from build123d import *

# Parameters (mm, degrees)
SKETCH1_W           = 81.5
SKETCH1_H           = 35
BOSS_EXTRUDE1_DEPTH = 3
SKETCH2_W           = 81.5
SKETCH2_H           = 35
BOSS_EXTRUDE2_DEPTH = 25.5


with BuildPart() as part:
    # Sketch1 → Boss-Extrude1 (new body)
    with BuildSketch(Plane(origin=(0, 0, 0), x_dir=(1, 0, 0), z_dir=(0, 1, 0))):
        with Locations((40.75, 17.5)):
            Rectangle(SKETCH1_W, SKETCH1_H)
    extrude(amount=BOSS_EXTRUDE1_DEPTH)

    # Sketch2 → Boss-Extrude2 (add)
    with BuildSketch(Plane(origin=(0, 3, 0), x_dir=(1, 0, 0), z_dir=(0, 1, 0))):
        with Locations((40.75, 17.5)):
            Rectangle(SKETCH2_W, SKETCH2_H)
        Polygon((79, 5), (79, 6.25), (77.899410911, 6.25), (77.899410911, 7.5), (79, 7.5), (79, 8.75), (77.899410911, 8.75), (77.899410911, 10), (79, 10), (79, 11.25), (77.899410911, 11.25), (77.899410911, 12.5), (79, 12.5), (79, 13.75), (77.899410911, 13.75), (77.899410911, 15), (79, 15), (79, 16.25), (77.899410911, 16.25), (77.899410911, 17.5), (79, 17.5), (79, 18.75), (77.899410911, 18.75), (77.899410911, 20), (79, 20), (79, 21.25), (77.899410911, 21.25), (77.899410911, 22.5), (79, 22.5), (79, 23.75), (77.899410911, 23.75), (77.899410911, 25), (79, 25), (79, 26.25), (77.899410911, 26.25), (77.899410911, 27.5), (79, 27.5), (79, 28.75), (77.899410911, 28.75), (77.899410911, 30), (79, 30), (79, 31.25), (77.899410911, 31.25), (77.899410911, 32.5), (3.600589089, 32.5), (3.600589089, 31.25), (2.5, 31.25), (2.5, 30), (3.600589089, 30), (3.600589089, 28.75), (2.5, 28.75), (2.5, 27.5), (3.600589089, 27.5), (3.600589089, 26.25), (2.5, 26.25), (2.5, 25), (3.600589089, 25), (3.600589089, 23.75), (2.5, 23.75), (2.5, 22.5), (3.600589089, 22.5), (3.600589089, 21.25), (2.5, 21.25), (2.5, 20), (3.600589089, 20), (3.600589089, 18.75), (2.5, 18.75), (2.5, 17.5), (3.600589089, 17.5), (3.600589089, 16.25), (2.5, 16.25), (2.5, 15), (3.600589089, 15), (3.600589089, 13.75), (2.5, 13.75), (2.5, 12.5), (3.600589089, 12.5), (3.600589089, 11.25), (2.5, 11.25), (2.5, 10), (3.600589089, 10), (3.600589089, 8.75), (2.5, 8.75), (2.5, 7.5), (3.600589089, 7.5), (3.600589089, 6.25), (2.5, 6.25), (2.5, 5), (3.600589089, 5), (3.600589089, 3.75), (2.5, 3.75), (2.5, 2.5), (79, 2.5), (79, 3.75), (77.899410911, 3.75), (77.899410911, 5), align=None, mode=Mode.SUBTRACT)
    extrude(amount=BOSS_EXTRUDE2_DEPTH)


solid = part.part
Could you check a few things on this model? Use its own coordinates, in mm. A direction names the side the tool comes from. Give positions to 0.01 mm unless a question says otherwise; leave off trailing zeros. Loops run counter-clockwise (first coordinate to the right, second up) from the corner with the lowest first, then second, coordinate; pieces in that order, holes last. Notation, with made-up numbers: M 51,71 L 89,71 A29 cw 89,93 Z; hole C 53.5,64.25 d4. An arc over 180 degrees is marked long. Answer as a JSON object with one key per item and string values.
Q1. If we mould it in two halves opening along X, with no side actions, what happens to faces 3 (the flat face through (81.5, 14, -17)), 4 (the flat face through (40, 16, -2.5)), 5 (the flat face through (40, 0, -18))? For each: pulls with the +X half, pulls with the -X half, needs draft (parallel to the pull), parting line crosses it, or undercut.
Values found:
{"face 3": "pulls with the +X half", "face 4": "undercut", "face 5": "needs draft"}
Q2. For P1, Ø8, axis at x = 61.5, z = -8, coming from the +Y side, with a flat end and sliding along its axis, tell me the tip position at first contact or that it passes through.
Values found:
{"P1": "stops at y = 3"}
Q3. If I drill on probe 1 along Z at (x, y) = (50.5, 22); probe 2 along X at (y, z) = (6.5, -20.5); probe 3 along Y at (x, z) = (15, -19.5), over which ranges is the centre line in solid material (lowest first)? Write a range as [from, to].
Values found:
{"probe 1": "z = [-35, -32.5], [-2.5, 0]", "probe 2": "x = [0, 2.5], [79, 81.5]", "probe 3": "y = [0, 3]"}
Q4. For faces 1 (the flat face through (41, 16, -32.5)), 2 (the flat face through (0, 14, -17)), which set-ups out of +Z, -Z, +X, -X, +Y, -Y let a thin tool reach every point of the face, with its end or its side?
Values found:
{"face 1": "+Y", "face 2": "+Z, -Z, -X, +Y, -Y"}
Q5. Suppose I cut it at A-A, the plane x = 53.5. List the corners of the cut face in (y, z) for me, plus the area to 4 significant figures.
Values found:
{"outline": "M 0,-35 L 28.5,-35 L 28.5,-32.5 L 3,-32.5 L 3,-2.5 L 28.5,-2.5 L 28.5,0 L 0,0 Z", "area": "232.5 mm²"}
